from build123d import *

# Parameters (mm, degrees)
FILLET1_R = 0.2


with BuildPart() as part:
    # BodySke → Base-Revolve (revolve)
    with BuildSketch(Plane.XY):
        Polygon((0, 0), (0, 3.75), (0.5, 4.25), (5, 4.25), (5, 2.5), (34.555, 2.5), (35, 2.055), (35, 0), align=None)
    revolve(axis=Axis((-31.75, 0, 0), (1, 0, 0)))

    # Fillet1
    fillet1_edges = [part.edges().sort_by_distance(p)[0] for p in [
        (5, -2.5, 0),
    ]]
    fillet(fillet1_edges, radius=FILLET1_R)


solid = part.part
Source: CAD feature listing. Evaluate the final solid. Frame: model axes, mm. A direction names the side the tool comes from. Coordinates: 2 decimals unless noted, no trailing zeros. Loops run counter-clockwise (first coordinate to the right, second up) from the corner with the lowest first, then second, coordinate; pieces in that order, holes last. Notation, with made-up numbers: (71.25, 40) -> (118.25, 40) arc R22 ccw to (118.25, 77) -> close; hole circle Ø1 at (20, -24). An arc over 180 degrees is marked (long way). Answer in a Markdown table with one row per item. Add a question column.
Q1. Section A-A on z = 0. Return the cut outline in (x, y) (3 decimals).
Q2. Contact query for flat-ended pins moving along their axis: pin 1 Ø5 at (x, z) = (19, 1.5) entering from +Y; pin 2 Ø1.5 at (x, z) = (15.5, 2.5) entering from -Y. Output: stop coordinate, or through.
Q3. Reachability of faces 1 (the face through (20.08, -0.54, -2.44)), 2 (the face through (0, 0, 0)) from +Z, -Z, +X, -X, +Y, -Y: full face, straight path, thin tool, end or side. Return the list, or none.
Q4. Ray query, line 1 along X through (y, z) = (-2.75, 2.25); line 2 along Z through (x, y) = (22, 0); line 3 along Z through (x, y) = (2.5, 3). Return the intervals inside material, ascending.
Q5. Section C-C on x = 19. Return the cut outline in (y, z).
Computed values:
| question | item | result |
|---|---|---|
| 1 | outline | (0, -3.75) -> (0.5, -4.25) -> (5, -4.25) -> (5, -2.7) arc R0.2 cw to (5.2, -2.5) -> (34.555, -2.5) -> (35, -2.055) -> (35, 2.055) -> (34.555, 2.5) -> (5.2, 2.5) arc R0.2 cw to (5, 2.7) -> (5, 4.25) -> (0.5, 4.25) -> (0, 3.75) -> close |
| 2 | pin 1 | stops at y = 2.5 |
| 2 | pin 2 | stops at y = -1.79 |
| 3 | face 1 | +X |
| 3 | face 2 | +Z, -Z, -X, +Y, -Y |
| 4 | line 1 | x = 0 to 5 |
| 4 | line 2 | z = -2.5 to 2.5 |
| 4 | line 3 | z = -3.01 to 3.01 |
| 5 | outline | circle Ø5 at (0, 0) |
